from build123d import *

# Parameters (mm, degrees)
SKETCH1_R           = 0.8
SKETCH1_R_2         = 3
BOSS_EXTRUDE1_DEPTH = 31
BOSS_EXTRUDE2_DEPTH = 1
SKETCH5_R           = 0.8
CUT_EXTRUDE3_DEPTH  = 1
SKETCH5_3_R         = 3
CUT_EXTRUDE4_DEPTH  = 1
CUT_EXTRUDE6_START  = -1
SKETCH6_W           = 28.997664588
SKETCH6_H           = 18.792631537
CUT_EXTRUDE6_DEPTH  = 104.494601352
SKETCH7_W           = 31
SKETCH7_H           = 56.017020421
CUT_EXTRUDE7_DEPTH  = 105.264671446
SKETCH8_R           = 1.5
CUT_EXTRUDE8_DEPTH  = 59.37205382


with BuildPart() as part:
    # Sketch1 → Boss-Extrude1 (new body)
    with BuildSketch(Plane(origin=(0, 0, 0), x_dir=(0, 0, -1), z_dir=(1, 0, 0))):
        with BuildLine():
            Line((27.520646447, 38.775594), (27.520646447, 55.275594))
            Line((27.520646447, 55.275594), (43.520646447, 55.275594))
            Line((43.520646447, 55.275594), (43.520646447, 38.775594))
            ThreePointArc((43.520646447, 38.775594), (35.520646447, 30.775594), (27.520646447, 38.775594))
        make_face()
        with Locations((35.520646447, 44.775594)):
            Circle(SKETCH1_R, mode=Mode.SUBTRACT)
        with Locations((41.515881392, 38.775594)):
            Circle(SKETCH1_R, mode=Mode.SUBTRACT)
        with Locations((35.520646447, 32.775594)):
            Circle(SKETCH1_R, mode=Mode.SUBTRACT)
        with Locations((29.515881392, 38.775594)):
            Circle(SKETCH1_R, mode=Mode.SUBTRACT)
        with Locations((35.520646447, 38.775594)):
            Circle(SKETCH1_R_2, mode=Mode.SUBTRACT)
    extrude(amount=BOSS_EXTRUDE1_DEPTH)

    # Sketch4 → Boss-Extrude2 (add)
    with BuildSketch(Plane(origin=(0, 55.275594, 0), x_dir=(1, 0, 0), z_dir=(0, 1, 0))):
        with BuildLine():
            Line((0, 43.520646447), (31, 43.520646447))
            Line((31, 43.520646447), (31, 65.088337856))
            Line((31, 65.088337856), (31, 81.236093118))
            ThreePointArc((31, 81.236093118), (15.5, 96.736093118), (0, 81.236093118))
            Line((0, 81.236093118), (0, 65.088337856))
            Line((0, 65.088337856), (0, 43.520646447))
        make_face()
    extrude(amount=-BOSS_EXTRUDE2_DEPTH)

    # Sketch5 → Cut-Extrude3 (cut)
    with BuildSketch(Plane.XZ.offset(-54.275594)):
        with Locations(Location((9.5, -81.236093118, 0), (0, 0, 270))):
            Circle(SKETCH5_R)
        with Locations(Location((15.5, -75.236093118, 0), (0, 0, 270))):
            Circle(SKETCH5_R)
        with Locations(Location((21.5, -81.236093118, 0), (0, 0, 270))):
            Circle(SKETCH5_R)
        with Locations(Location((15.5, -87.236093118, 0), (0, 0, 270))):
            Circle(SKETCH5_R)
    extrude(amount=-CUT_EXTRUDE3_DEPTH, mode=Mode.SUBTRACT)

    # Sketch5_3 → Cut-Extrude4 (cut)
    with BuildSketch(Plane.XZ.offset(-54.275594)):
        with Locations(Location((15.5, -81.236093118, 0), (0, 0, 270))):
            Circle(SKETCH5_3_R)
    extrude(amount=-CUT_EXTRUDE4_DEPTH, mode=Mode.SUBTRACT)

    # Sketch6 → Cut-Extrude6 (cut, through all)
    with BuildSketch(Plane(origin=(0, 55.275594, 0), x_dir=(1, 0, 0), z_dir=(0, 1, 0)).offset(CUT_EXTRUDE6_START)):
        with Locations((15.5, 35.520646447)):
            Rectangle(SKETCH6_W, SKETCH6_H)
    extrude(amount=-CUT_EXTRUDE6_DEPTH, mode=Mode.SUBTRACT)

    # Sketch7 → Cut-Extrude7 (cut, through all)
    with BuildSketch(Plane.XZ.offset(-54.275594)):
        with Locations((15.5, -71.529156658)):
            Rectangle(SKETCH7_W, SKETCH7_H)
    extrude(amount=-CUT_EXTRUDE7_DEPTH, mode=Mode.SUBTRACT)

    # Sketch8 → Cut-Extrude8 (cut, through all)
    with BuildSketch(Plane.XZ.offset(-54.275594)):
        with Locations(Location((7.75, -35.520646447, 0), (0, 0, 270))):
            Circle(SKETCH8_R)
        with Locations(Location((23.25, -35.520646447, 0), (0, 0, 270))):
            Circle(SKETCH8_R)
    extrude(amount=-CUT_EXTRUDE8_DEPTH, mode=Mode.SUBTRACT)


solid = part.part
Verification items for the finished model (mm, model axes). A direction names the side the tool comes from. Coordinates: 2 decimals unless noted, no trailing zeros. Order: outer loops, then holes, each group sorted by start corner. A loop starts at its lowest first (then second) coordinate and runs counter-clockwise, first axis right, second up. Notation, with made-up numbers: (84.5, 35) -> (139.5, 35) arc R31 cw to (139.5, 68) -> close; hole circle Ø9 at (73.25, 49). An arc over 180 degrees is marked (long way). Put each result on its own line as item: value. Start each with the question number.
1. Cross-section at A-A, the plane x = 23.25. Record the boundary of the cut face in (y, z), then the cut area to 3 significant figures.
2. Cross-section at B-B, the plane y = 34.25. Record the boundary of the cut face in (x, z), then the cut area to 3 significant figures.
3. Cross-section at D-D, the plane z = -33.5. Record the boundary of the cut face in (x, y).
4. Cross-section at C-C, the plane z = -37.5. Record the boundary of the cut face in (x, y).
5. Material ranges on L1, parallel to X at y = 36.5, z = -39.5; L2, parallel to Y at x = 28, z = -38.5, recorded low to high. Write a range as [from, to].
6. Mould release check, pull along X, two halves, no side actions. Record for faces 3 (the flat face through (1.001, 43, -35)), 4 (the flat face through (31, 43, -35)), 5 (the cylindrical face through (0.49, 38.07, -41.89)), 6 (the flat face through (0, 43, -36)): released by +X, released by -X, zero draft, split by the parting line, or undercut.
7. Access from +Z, -Z, +X, -X, +Y, -Y to the whole of each face (thin tool, end or side, straight path). Record for faces 1 (the flat face through (29.999, 43, -35)), 2 (the cylindrical face through (30.49, 39.68, -38.38)).
8. Go/stop test with a flat-tipped pin: pin 1 Ø8 at (x, z) = (14.5, -39) entering from -Y. Record where the tip stops, or that it passes through.
Computed:
1. outline: (54.28, -43.52) -> (55.28, -43.52) -> (55.28, -37.02) -> (54.28, -37.02) -> close; (54.28, -34.02) -> (55.28, -34.02) -> (55.28, -27.52) -> (54.28, -27.52) -> close
1. area: 13.0 mm2
2. outline: (0, -42.12) -> (1, -42.12) -> (1, -28.92) -> (0, -28.92) -> close; (30, -42.12) -> (31, -42.12) -> (31, -28.92) -> (30, -28.92) -> close
2. area: 26.4 mm2
3. outline: (0, 31.03) -> (1, 31.03) -> (1, 36.56) -> (0, 36.56) -> close; (0, 40.99) -> (1, 40.99) -> (1, 54.28) -> (30, 54.28) -> (30, 40.99) -> (31, 40.99) -> (31, 55.28) -> (0, 55.28) -> close; (30, 31.03) -> (31, 31.03) -> (31, 36.56) -> (30, 36.56) -> close
4. outline: (0, 31.02) -> (1, 31.02) -> (1, 36.52) -> (0, 36.52) -> close; (0, 41.03) -> (1, 41.03) -> (1, 54.28) -> (30, 54.28) -> (30, 41.03) -> (31, 41.03) -> (31, 55.28) -> (0, 55.28) -> close; (30, 31.02) -> (31, 31.02) -> (31, 36.52) -> (30, 36.52) -> close
5. L1: [0, 1], [30, 31]
5. L2: [54.28, 55.28]
6. face 3: undercut
6. face 4: released by +X
6. face 5: zero draft
6. face 6: released by -X
7. face 1: +Z, -Z, -Y
7. face 2: +X, -X
8. pin 1: y = 54.28
